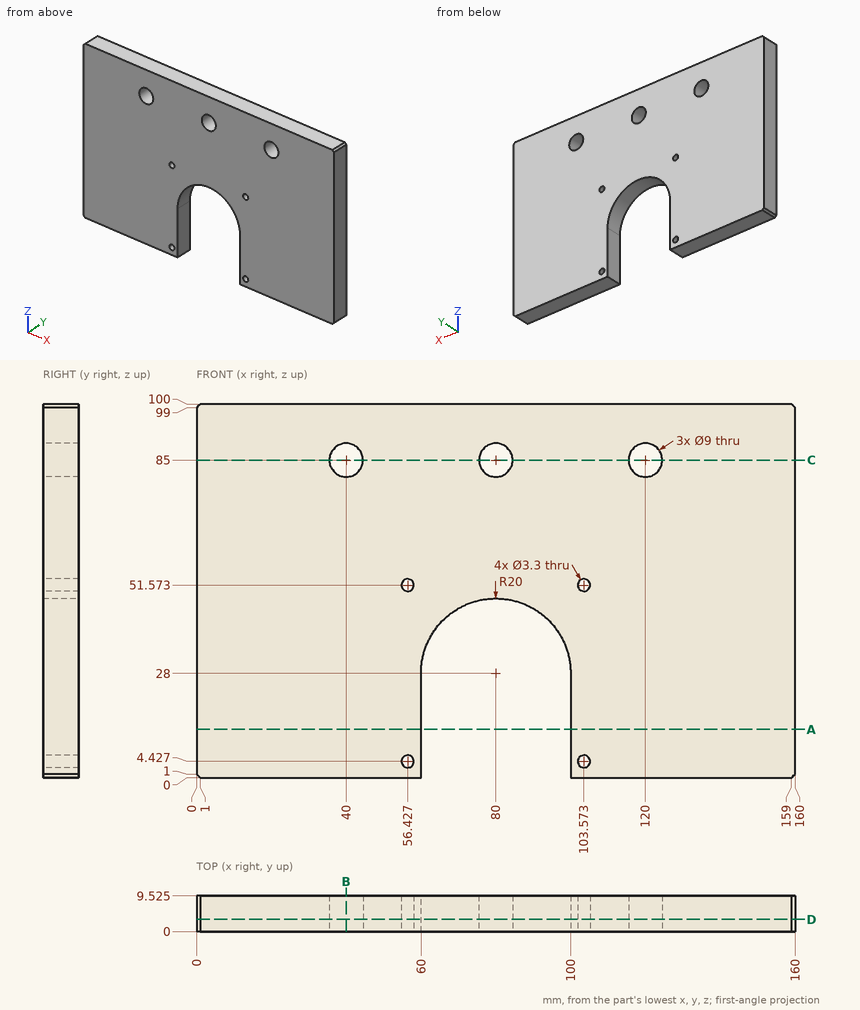
Check sheet for the drawn part. Datum: minimum x, y, z corner. Units: mm. Round coordinates to 2 decimals unless told otherwise and drop trailing zeros. Write each loop counter-clockwise with the first axis right and the second up, starting at its lowest first coordinate (ties: lowest second). Pieces come first, ordered by that corner, then holes. Notation, with made-up numbers: (78.25, 18.5) - (91.25, 18.5) arc R19 ccw to (91.25, 33.5) - close; hole circle Ø4 at (30.25, 54.25). An arc over 180 degrees is marked (long way). Return JSON: item names as keys, results as strings.
Q1. Depth check by flat-ended pin: P1, Ø5.5, axis at x = 80, z = 85, coming from the +Y side; P2, Ø4, axis at x = 78, y = 4, coming from the -Z side. Enter the tip coordinate at first touch or a pass-through.
Returned:
{"P1": "passes through", "P2": "stops at z = 47.6"}
Q2. Cross-section at D-D (y = 3.25). Record the boundary of the cut face in (x, z).
Returned:
{"outline": "(0, 1) - (1, 0) - (60, 0) - (60, 28) arc R20 cw to (100, 28) - (100, 0) - (159, 0) - (160, 1) - (160, 99) - (159, 100) - (1, 100) - (0, 99) - close; hole circle Ø9 at (40, 85); hole circle Ø3.3 at (56.43, 4.43); hole circle Ø3.3 at (56.43, 51.57); hole circle Ø9 at (80, 85); hole circle Ø3.3 at (103.57, 4.43); hole circle Ø3.3 at (103.57, 51.57); hole circle Ø9 at (120, 85)"}
Q3. Scan lines: L1, parallel to X at y = 5.5, z = 85; L2, parallel to Z at x = 120, y = 4; L3, parallel to X at y = 2.5, z = 83.5. Record each from-to range of solid material in increasing order. Write a range as from..to.
Returned:
{"L1": "x = 0..35.5, 44.5..75.5, 84.5..115.5, 124.5..160", "L2": "z = 0..80.5, 89.5..100", "L3": "x = 0..35.76, 44.24..75.76, 84.24..115.76, 124.24..160"}
Q4. Cross-section at B-B (x = 40). Record the boundary of the cut face in (y, z) (3 decimals).
Returned:
{"outline": "(0, 0) - (9.525, 0) - (9.525, 80.5) - (0, 80.5) - close; (0, 89.5) - (9.525, 89.5) - (9.525, 100) - (0, 100) - close"}
Q5. Cross-section at C-C (z = 85). Record the boundary of the cut face in (x, y) (3 decimals).
Returned:
{"outline": "(0, 0) - (35.5, 0) - (35.5, 9.525) - (0, 9.525) - close; (44.5, 0) - (75.5, 0) - (75.5, 9.525) - (44.5, 9.525) - close; (84.5, 0) - (115.5, 0) - (115.5, 9.525) - (84.5, 9.525) - close; (124.5, 0) - (160, 0) - (160, 9.525) - (124.5, 9.525) - close"}
Q6. Cross-section at A-A (z = 13). Record the boundary of the cut face in (x, y) (3 decimals), then the cut area to 3 significant figures.
Returned:
{"outline": "(0, 0) - (60, 0) - (60, 9.525) - (0, 9.525) - close; (100, 0) - (160, 0) - (160, 9.525) - (100, 9.525) - close", "area": "1,140 mm²"}
